Source: CAD feature listing. Evaluate the final solid. Frame: model axes, mm. Face numbers are marked on the shaded views. A direction names the side the tool comes from. Round coordinates to 2 decimals unless told otherwise and drop trailing zeros. Write each loop counter-clockwise with the first axis right and the second up, starting at its lowest first coordinate (ties: lowest second). Pieces come first, ordered by that corner, then holes. Notation, with made-up numbers: M 87,8.25 L 112,8.25 A33 cw 112,41.25 Z; hole C -1.5,1 d6. An arc over 180 degrees is marked long. Use a Markdown table: item, result.
Autodesk Inventor part; units mm, degrees
ref_plane "YZ Plane" through (0, 0, 0) normal (1, 0, 0) x (0, 1, 0)
ref_plane "XZ Plane" through (0, 0, 0) normal (0, 1, 0) x (-1, 0, 0)
ref_plane "XY Plane" through (0, 0, 0) normal (0, 0, 1) x (1, 0, 0)
sketch "Sketch1" plane through (0, 0, 0) normal (1, 0, 0) x (0, 1, 0)
  line L0 (0, 0) -> (-152.4, 0)
  line L1 (-152.4, 0) -> (-152.4, 3.175)
  line L2 (-152.4, 3.175) -> (0, 3.175)
  line L3 (0, 3.175) -> (0, 0)
  dimension "d0" = 152.4
  dimension "d1" = 3.175
extrude "Extrusion1" add sketch "Sketch1" along normal blind 400.05
sketch "Sketch2" plane through (0, 0, 0) normal (-1, 0, 0) x (0, 0, 1)
  line L0 (0, 0) -> (3.175, 0)
  line L1 (3.175, 0) -> (-34.7333, 3.8172)
  line L2 (-34.7333, 3.8172) -> (-37.2781, -21.455)
  line L3 (-37.2781, -21.455) -> (-21.3975, -124.5257)
  line L4 (-21.3975, -124.5257) -> (3.175, -127)
  line L5 (3.175, -127) -> (3.175, 0)
  line L6 (0, -152.4) -> (0, 0)
  circle A0 centre (-8.255, -113.7628) radius 3.175
  line L7 (-21.3975, -124.5257) -> (3.175, -120.7397) construction
  line L8 (3.175, 0) -> (3.175, -152.4)
  circle A1 centre (-23.3696, -10.0913) radius 3.175
  dimension "d4" = 25.4
  dimension "d5" = 95.75
  dimension "d6" = 38.1
  dimension "d7" = 127
  dimension "d8" = 104.2869
  dimension "d9" = 6.35
  dimension "d11" = 11.43
  dimension "d12" = 8.636
  dimension "d15" = 12.7
  dimension "d16" = 6.35
  dimension "d17" = 12.7
extrude "Extrusion3" add sketch "Sketch2" along normal blind 3.175
ref_plane "Work Plane1" through (200.025, 0, 0) normal (-1, 0, 0) x (0, 0, 1)
mirror "Mirror1" about plane through (200.025, 0, 0) normal (-1, 0, 0) of "Extrusion3"
properties part number "15102898-16-P-0215" material "Aluminum 6061"
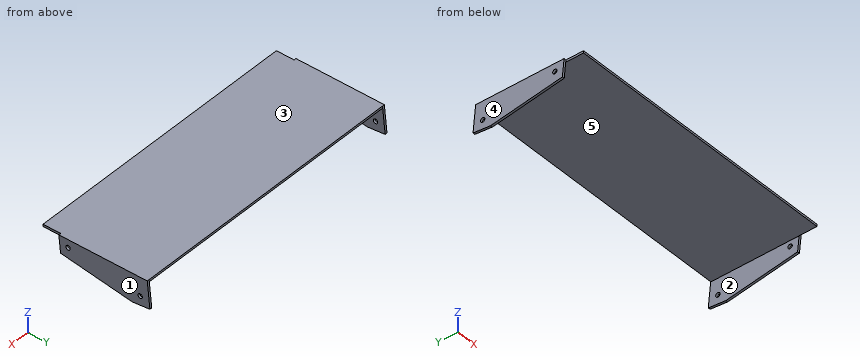
Q1. Section A-A on y = -102. Return loops of the section in (x, z) (3 decimals), plus the area to 3 significant figures.
Results are:
| item | result |
|---|---|
| outline | M -3.175,-24.868 L 0,-24.868 L 0,0 L 400.05,0 L 400.05,-24.868 L 403.225,-24.868 L 403.225,3.175 L -3.175,3.175 Z |
| area | 1,450 mm^2 |
Q2. Section B-B on x = 42. Return loops of the section in (y, z) (3 decimals).
Results are:
| item | result |
|---|---|
| outline | M -152.4,0 L 0,0 L 0,3.175 L -152.4,3.175 Z |
Q3. Line query: L1, parallel to X at y = -28.5, z = -3 (3 decimals); L2, parallel to Z at x = 126.5, y = -46.5 (3 decimals); L3, parallel to Y at x = 219.5, z = 1. Output: solid intervals per line, ascending.
Results are:
| item | result |
|---|---|
| L1 | -3.175 to 0, 400.05 to 403.225 |
| L2 | 0 to 3.175 |
| L3 | -152.4 to 0 |
Q4. Mould query, pull axis X, two halves, no side actions, for the marked faces 3, 4 and 5. Classes: +X half, -X half, draft (parallel to the pull), parting line (faces both ways), or undercut.
Results are:
| item | result |
|---|---|
| face 3 | draft |
| face 4 | -X half |
| face 5 | undercut |
Q5. Reachability of the marked faces 1 and 2 from +Z, -Z, +X, -X, +Y, -Y: full face, straight path, thin tool, end or side. Return the list, or none.
Results are:
| item | result |
|---|---|
| face 1 | +Z, -Z, +X, +Y, -Y |
| face 2 | -Z, +Y, -Y |
Q6. Section C-C on y = -72.5. Return loops of the section in (x, z) (3 decimals).
Results are:
| item | result |
|---|---|
| outline | M -3.175,-29.413 L 0,-29.413 L 0,0 L 400.05,0 L 400.05,-29.413 L 403.225,-29.413 L 403.225,3.175 L -3.175,3.175 Z |
Q7. First-contact query: pin 1 Ø4 at (y, z) = (-10.09, -23.37) entering from +X; pin 2 Ø2.5 at (y, z) = (-141.5, 1) entering from +X; pin 3 Ø4 at (x, y) = (325.5, -19.5) entering from -Z; pin 4 Ø3.5 at (x, z) = (190, 2) entering from +Y. Flat tips, straight axial feed; report the tip coordinate or a pass-through.
Results are:
| item | result |
|---|---|
| pin 1 | through |
| pin 2 | x = 400.05 |
| pin 3 | z = 0 |
| pin 4 | y = 0 |
